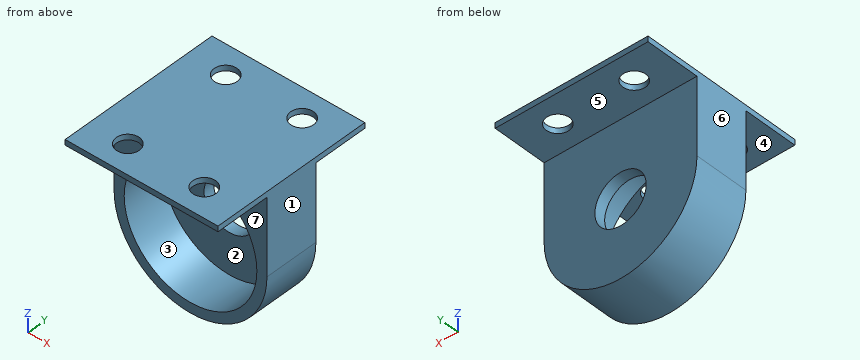
from build123d import *

# Parameters (mm, degrees)
SKETCH1_R                   = 4.7
BOSS_EXTRUDE1_DEPTH         = 10
SKETCH2_W                   = 28
SKETCH2_H                   = 30
BOSS_EXTRUDE2_DEPTH         = 1
TAP_DRILL_FOR_M5X0_8_TAP1_D = 4.2
SKETCH5_R                   = 12.15
SKETCH5_R_2                 = 4.7
CUT_EXTRUDE1_DEPTH          = 8


with BuildPart() as part:
    # Sketch1 → Boss-Extrude1 (new body)
    with BuildSketch(Plane(origin=(0, 0, 0), x_dir=(1, 0, 0), z_dir=(0, 1, 0))):
        with BuildLine():
            Line((0, 1.238241861), (0, 15.238241861))
            ThreePointArc((0, 15.238241861), (-14, 29.238241861), (-28, 15.238241861))
            Line((-28, 15.238241861), (-28, 1.238241861))
            Line((-28, 1.238241861), (0, 1.238241861))
        make_face()
        with Locations(Location((-14, 15.238241861, 0), (0, 0, 270))):
            Circle(SKETCH1_R, mode=Mode.SUBTRACT)
    extrude(amount=BOSS_EXTRUDE1_DEPTH)

    # Sketch2 → Boss-Extrude2 (add)
    with BuildSketch(Plane.XY.offset(-1.238241861)):
        with Locations((-14, 5)):
            Rectangle(SKETCH2_W, SKETCH2_H)
    extrude(amount=BOSS_EXTRUDE2_DEPTH)

    # Tap Drill for M5x0.8 Tap1 (through all)
    with Locations(Plane(origin=(0, 0, -1.238241861), x_dir=(-1, 0, 0), z_dir=(0, 0, -1))):
        with Locations((7, 15), (21, 15), (7, -5), (21, -5)):
            Hole(TAP_DRILL_FOR_M5X0_8_TAP1_D / 2)

    # Sketch5 → Cut-Extrude1 (cut)
    with BuildSketch(Plane.XZ):
        with Locations(Location((-14, -15.238241861, 0), (0, 0, 270))):
            Circle(SKETCH5_R)
        with Locations(Location((-14, -15.238241861, 0), (0, 0, 270))):
            Circle(SKETCH5_R_2, mode=Mode.SUBTRACT)
    extrude(amount=-CUT_EXTRUDE1_DEPTH, mode=Mode.SUBTRACT)


solid = part.part
Verification items for the finished model (mm, model axes). Face numbers are marked on the shaded views. A direction names the side the tool comes from. Give positions to 0.01 mm unless a question says otherwise; leave off trailing zeros. Write each loop counter-clockwise with the first axis right and the second up, starting at its lowest first coordinate (ties: lowest second). Pieces come first, ordered by that corner, then holes.
(1) Cross-section at D-D (y = 5). Enter the section's corners in (x, z), plus the area to 3 significant figures.
(2) Gauge pin test, flat ends, axial feed: pin 1 (3 mm diameter, centred on x = -15, y = 13.5, fed in from -Z); pin 2 (10 mm diameter, centred on x = -3, z = -7.5, fed in from +Y). Record the tip position at first contact, or that the pin passes through.
(3) Cross-section at B-B (x = -6.75). Enter the section's corners in (y, z).
(4) Cross-section at A-A (y = -5). Enter the section's corners in (x, z).
(5) Cross-section at C-C (x = -14). Enter the section's corners in (y, z).
(6) Mould release check, pull along Z, two halves, no side actions. Record for the marked faces 1, 2, 3 and 4: +Z half, -Z half, draft (parallel to the pull), parting line (faces both ways), or undercut.
(7) Material ranges on line 1 (Y direction, x = -21, z = -0.65); line 2 (Y direction, x = -20.25, z = -13.5); line 3 (Z direction, x = -2, y = 13.75), recorded low to high.
(8) Access from +Z, -Z, +X, -X, +Y, -Y to the whole of each face (thin tool, end or side, straight path). Record for the marked faces 5, 6 and 7.
Worked out:
1. outline: (-28, -15.24) arc R14 ccw to (0, -15.24) - (0, -0.24) - (-28, -0.24) - close; hole circle Ø24.3 at (-14, -15.24)
1. area: 264 mm2
2. pin 1: stops at z = -1.24
2. pin 2: stops at y = 10
3. outline: (-10, -1.24) - (-7.09, -1.24) - (-7.09, -0.24) - (-10, -0.24) - close; (-2.91, -1.24) - (0, -1.24) - (0, -5.49) - (8, -5.49) - (8, -24.99) - (0, -24.99) - (0, -27.21) - (10, -27.21) - (10, -1.24) - (12.91, -1.24) - (12.91, -0.24) - (-2.91, -0.24) - close; (17.09, -1.24) - (20, -1.24) - (20, -0.24) - (17.09, -0.24) - close
4. outline: (-28, -1.24) - (-23.1, -1.24) - (-23.1, -0.24) - (-28, -0.24) - close; (-18.9, -1.24) - (-9.1, -1.24) - (-9.1, -0.24) - (-18.9, -0.24) - close; (-4.9, -1.24) - (0, -1.24) - (0, -0.24) - (-4.9, -0.24) - close
5. outline: (-10, -1.24) - (0, -1.24) - (0, -3.09) - (8, -3.09) - (8, -10.54) - (10, -10.54) - (10, -1.24) - (20, -1.24) - (20, -0.24) - (-10, -0.24) - close; (0, -29.24) - (10, -29.24) - (10, -19.94) - (8, -19.94) - (8, -27.39) - (0, -27.39) - close
6. face 1: draft
6. face 2: undercut
6. face 3: undercut
6. face 4: -Z half
7. line 1: y = -10 to -7.1, -2.9 to 12.9, 17.1 to 20
7. line 2: y = 8 to 10
7. line 3: z = -1.24 to -0.24
8. face 5: -Z, +X, -X, +Y
8. face 6: +Z, -Z, -X, +Y, -Y
8. face 7: -Z, +X, -X, -Y
